Source: CAD feature listing. Evaluate the final solid. Frame: model axes, mm. Face numbers are marked on the shaded views. A direction names the side the tool comes from. Give positions to 0.01 mm unless a question says otherwise; leave off trailing zeros. Write each loop counter-clockwise with the first axis right and the second up, starting at its lowest first coordinate (ties: lowest second). Pieces come first, ordered by that corner, then holes. Notation, with made-up numbers: (45.5, 5) - (86.5, 5) arc R24 ccw to (86.5, 29) - close; hole circle Ø5 at (-40, 43.25). An arc over 180 degrees is marked (long way). One line per question, with ' | ' between items. Start each with the question number.
(1) Section D-D, the plane z = 5.75. Return loops of the section in (x, y) (3 decimals), plus the area to 3 significant figures.
(2) Section B-B, the plane x = 0. Return loops of the section in (y, z) (3 decimals).
(3) Section A-A, the plane z = 9.5. Return loops of the section in (x, y) (3 decimals), plus the area to 3 significant figures.
(4) Section C-C, the plane y = -9.5. Return loops of the section in (x, z), plus the area to 3 significant figures.
(5) Access query for the marked faces 5, 6 and 7. Directions: +Z, -Z, +X, -X, +Y, -Y. A direction counts if a zero-diameter tool reaches every point of the face in a straight line with its end or side. Return the directions, or none.
(6) Pin query (flat end, axial travel): pin 1 (1 mm diameter, centred on y = -17.5, z = -3.5, fed in from +X); pin 2 (1 mm diameter, centred on y = -17.5, z = -1.5, fed in from -X); pin 3 (0.5 mm diameter, centred on x = 2, z = -1.5, fed in from +Y) (3 decimals). Return the tip coordinate at first contact, or that it passes through.
(7) Draft query along Y for the marked faces 1, 2, 3 and 4. Return one class per face: +Y half, -Y half, draft (parallel to the pull), parting line (faces both ways), or undercut.
(8) Ray query, line 1 (Y direction, x = 0, z = 3.5) (3 decimals); line 2 (Y direction, x = 0, z = 4) (3 decimals); line 3 (X direction, y = -8, z = 6.75). Return the intervals inside material, ascending. Write a range as [from, to].
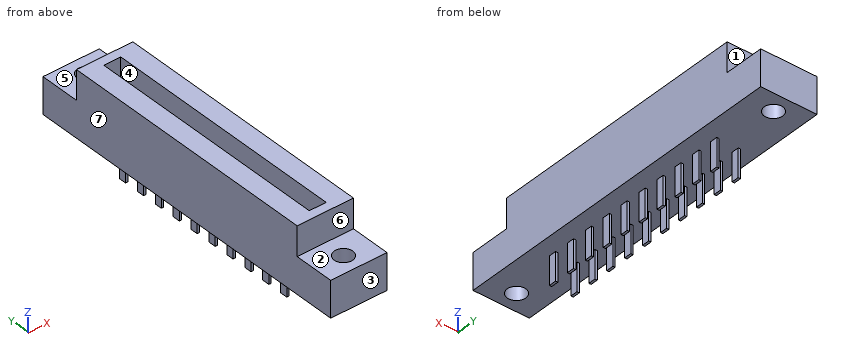
```python
from build123d import *

# Parameters (mm, degrees)
SKETCH_1_W          = 10
SKETCH_1_H          = 61.2
EXTRUDE_1_DEPTH     = 6.4
SKETCH_2_W          = 10
SKETCH_2_H          = 46.93
EXTRUDE_2_DEPTH     = 5.2
SKETCH_3_R          = 1.65
CUT_EXTRUDE_1_DEPTH = 15.3
SKETCH_4_W          = 0.41
SKETCH_4_H          = 1.3
EXTRUDE_3_DEPTH     = 5
SKETCH_5_W          = 3
SKETCH_5_H          = 43.7
CUT_EXTRUDE_2_DEPTH = 8


with BuildPart() as part:
    # 草图1 → 拉伸1 (new body)
    with BuildSketch(Plane.XY):
        Rectangle(SKETCH_1_W, SKETCH_1_H)
    extrude(amount=EXTRUDE_1_DEPTH)

    # 草图2 → 拉伸2 (add)
    with BuildSketch(Plane.XY.offset(6.4)):
        Rectangle(SKETCH_2_W, SKETCH_2_H)
    extrude(amount=EXTRUDE_2_DEPTH)

    # 草图3 → 切除-拉伸1 (cut)
    with BuildSketch(Plane.XY.offset(6.4)):
        with Locations((0, 27.335)):
            Circle(SKETCH_3_R)
        with Locations((0, -27.335)):
            Circle(SKETCH_3_R)
    extrude(amount=-CUT_EXTRUDE_1_DEPTH, mode=Mode.SUBTRACT)

    # 草图4 → 拉伸3 (add)
    with BuildSketch(Plane(origin=(0, 0, 0), x_dir=(-1, 0, 0), z_dir=(0, 0, -1))):
        with Locations((-1.905, 1.905)):
            Rectangle(SKETCH_4_W, SKETCH_4_H)
        with Locations((1.905, 1.905)):
            Rectangle(SKETCH_4_W, SKETCH_4_H)
        with Locations((-1.905, 5.715)):
            Rectangle(SKETCH_4_W, SKETCH_4_H)
        with Locations((1.905, 5.715)):
            Rectangle(SKETCH_4_W, SKETCH_4_H)
        with Locations((-1.905, 9.525)):
            Rectangle(SKETCH_4_W, SKETCH_4_H)
        with Locations((1.905, 9.525)):
            Rectangle(SKETCH_4_W, SKETCH_4_H)
        with Locations((-1.905, 13.335)):
            Rectangle(SKETCH_4_W, SKETCH_4_H)
        with Locations((1.905, 13.335)):
            Rectangle(SKETCH_4_W, SKETCH_4_H)
        with Locations((-1.905, 17.145)):
            Rectangle(SKETCH_4_W, SKETCH_4_H)
        with Locations((1.905, 17.145)):
            Rectangle(SKETCH_4_W, SKETCH_4_H)
        with Locations((-1.905, -1.905)):
            Rectangle(SKETCH_4_W, SKETCH_4_H)
        with Locations((1.905, -1.905)):
            Rectangle(SKETCH_4_W, SKETCH_4_H)
        with Locations((-1.905, -5.715)):
            Rectangle(SKETCH_4_W, SKETCH_4_H)
        with Locations((1.905, -5.715)):
            Rectangle(SKETCH_4_W, SKETCH_4_H)
        with Locations((-1.905, -9.525)):
            Rectangle(SKETCH_4_W, SKETCH_4_H)
        with Locations((1.905, -9.525)):
            Rectangle(SKETCH_4_W, SKETCH_4_H)
        with Locations((-1.905, -13.335)):
            Rectangle(SKETCH_4_W, SKETCH_4_H)
        with Locations((1.905, -13.335)):
            Rectangle(SKETCH_4_W, SKETCH_4_H)
        with Locations((-1.905, -17.145)):
            Rectangle(SKETCH_4_W, SKETCH_4_H)
        with Locations((1.905, -17.145)):
            Rectangle(SKETCH_4_W, SKETCH_4_H)
    extrude(amount=EXTRUDE_3_DEPTH)

    # 草图5 → 切除-拉伸2 (cut)
    with BuildSketch(Plane.XY.offset(11.6)):
        Rectangle(SKETCH_5_W, SKETCH_5_H)
    extrude(amount=-CUT_EXTRUDE_2_DEPTH, mode=Mode.SUBTRACT)


solid = part.part
```
Check sheet entries:
1) outline: (-5, -30.6) - (5, -30.6) - (5, 30.6) - (-5, 30.6) - close; hole circle Ø3.3 at (0, -27.335); hole circle Ø3.3 at (0, 27.335); hole (-1.5, -21.85) - (1.5, -21.85) - (1.5, 21.85) - (-1.5, 21.85) - close | area: 464 mm²
2) outline: (-30.6, 0) - (-28.985, 0) - (-28.985, 6.4) - (-30.6, 6.4) - close; (-25.685, 0) - (25.685, 0) - (25.685, 6.4) - (23.465, 6.4) - (23.465, 11.6) - (21.85, 11.6) - (21.85, 3.6) - (-21.85, 3.6) - (-21.85, 11.6) - (-23.465, 11.6) - (-23.465, 6.4) - (-25.685, 6.4) - close; (28.985, 0) - (30.6, 0) - (30.6, 6.4) - (28.985, 6.4) - close
3) outline: (-5, -23.465) - (5, -23.465) - (5, 23.465) - (-5, 23.465) - close; hole (-1.5, -21.85) - (1.5, -21.85) - (1.5, 21.85) - (-1.5, 21.85) - close | area: 338 mm²
4) outline: (-5, 0) - (-2.11, 0) - (-2.11, -5) - (-1.7, -5) - (-1.7, 0) - (1.7, 0) - (1.7, -5) - (2.11, -5) - (2.11, 0) - (5, 0) - (5, 11.6) - (1.5, 11.6) - (1.5, 3.6) - (-1.5, 3.6) - (-1.5, 11.6) - (-5, 11.6) - close | area: 96.1 mm²
5) face 5: +Z, +X, -X, +Y | face 6: +Z, +X, -X, -Y | face 7: +Z, -Z, -X, +Y, -Y
6) pin 1: x = 2.11 | pin 2: x = -2.11 | pin 3: y = 17.795
7) face 1: +Y half | face 2: draft | face 3: -Y half | face 4: undercut
8) line 1: [-30.6, -28.985], [-25.685, 25.685], [28.985, 30.6] | line 2: [-30.6, -28.985], [-25.685, -21.85], [21.85, 25.685], [28.985, 30.6] | line 3: [-5, -1.5], [1.5, 5]
